from build123d import *

# Parameters (mm, degrees)
CROQUIS1_R              = 6.35
SALIENTE_EXTRUIR1_DEPTH = 6.35
CROQUIS4_W              = 4.7625
CROQUIS4_H              = 50.8
CORTAR_EXTRUIR1_DEPTH   = 3.175


with BuildPart() as part:
    # Croquis1 → Saliente-Extruir1 (new body)
    with BuildSketch(Plane(origin=(0, 0, 0), x_dir=(1, 0, 0), z_dir=(0, 1, 0))):
        with BuildLine():
            Line((35.8, -25.4), (50.8, 0))
            Line((50.8, 0), (35.8, 25.4))
            Line((35.8, 25.4), (-100, 25.4))
            Line((-100, 25.4), (-144.746813481, 47.731727951))
            ThreePointArc((-144.746813481, 47.731727951), (-149.357530471, 48.146831931), (-153.024774803, 45.321528145))
            Line((-153.024774803, 45.321528145), (-165, 25.4))
            Line((-165, 25.4), (-165, -25.4))
            Line((-165, -25.4), (-214.07384035, -47.316891892))
            Line((-214.07384035, -47.316891892), (-147.685890016, -48.399156383))
            ThreePointArc((-147.685890016, -48.399156383), (-146.176180179, -48.24234101), (-144.746813481, -47.731727951))
            Line((-144.746813481, -47.731727951), (-100, -25.4))
            Line((-100, -25.4), (35.8, -25.4))
        make_face()
        with Locations(Location((0, 0, 0), (0, 0, 270))):
            Circle(CROQUIS1_R, mode=Mode.SUBTRACT)
        with Locations(Location((-150, 0, 0), (0, 0, 270))):
            Circle(CROQUIS1_R, mode=Mode.SUBTRACT)
        with BuildLine():
            Line((-118.545100716, 27.558404082), (-142.329198773, 39.428299747))
            ThreePointArc((-142.329198773, 39.428299747), (-146.939915763, 39.843403727), (-150.607160095, 37.018099941))
            Line((-150.607160095, 37.018099941), (-157.742389512, 25.148204276))
            ThreePointArc((-157.742389512, 25.148204276), (-157.827056347, 18.750312726), (-152.3, 15.526676131))
            Line((-152.3, 15.526676131), (-121.380672526, 15.526676131))
            ThreePointArc((-121.380672526, 15.526676131), (-115.199998109, 20.420048603), (-118.545100716, 27.558404082))
        make_face(mode=Mode.SUBTRACT)
        with BuildLine():
            Line((-118.545100716, -27.558404082), (-142.329198773, -39.428299747))
            ThreePointArc((-142.329198773, -39.428299747), (-146.939915763, -39.843403727), (-150.607160095, -37.018099941))
            Line((-150.607160095, -37.018099941), (-157.742389512, -25.148204276))
            ThreePointArc((-157.742389512, -25.148204276), (-157.827056347, -18.750312726), (-152.3, -15.526676131))
            Line((-152.3, -15.526676131), (-121.380672526, -15.526676131))
            ThreePointArc((-121.380672526, -15.526676131), (-115.199998109, -20.420048603), (-118.545100716, -27.558404082))
        make_face(mode=Mode.SUBTRACT)
        with BuildLine():
            Line((-130, 6.35), (-110, 6.35))
            ThreePointArc((-110, 6.35), (-103.65, 0), (-110, -6.35))
            Line((-110, -6.35), (-130, -6.35))
            ThreePointArc((-130, -6.35), (-136.35, 0), (-130, 6.35))
        make_face(mode=Mode.SUBTRACT)
        with BuildLine():
            Line((-56.70082756, -7.67562673), (-77.066937646, 8.064222026))
            ThreePointArc((-77.066937646, 8.064222026), (-83.748665223, 8.739846385), (-87.3, 3.039848756))
            Line((-87.3, 3.039848756), (-87.3, -12.7))
            ThreePointArc((-87.3, -12.7), (-85.440128061, -17.190128061), (-80.95, -19.05))
            Line((-80.95, -19.05), (-60.583889913, -19.05))
            ThreePointArc((-60.583889913, -19.05), (-54.57442778, -14.751551819), (-56.70082756, -7.67562673))
        make_face(mode=Mode.SUBTRACT)
        with BuildLine():
            Line((-57.963298738, 19.05), (-38.1, 19.05))
            ThreePointArc((-38.1, 19.05), (-33.609871939, 17.190128061), (-31.75, 12.7))
            Line((-31.75, 12.7), (-31.75, -2.651253459))
            ThreePointArc((-31.75, -2.651253459), (-35.301334777, -8.351251089), (-41.983062354, -7.67562673))
            Line((-41.983062354, -7.67562673), (-61.846361092, 7.67562673))
            ThreePointArc((-61.846361092, 7.67562673), (-63.972760872, 14.751551819), (-57.963298738, 19.05))
        make_face(mode=Mode.SUBTRACT)
    extrude(amount=SALIENTE_EXTRUIR1_DEPTH)

    # Croquis4 → Cortar-Extruir1 (cut)
    with BuildSketch(Plane(origin=(0, 6.35, 0), x_dir=(1, 0, 0), z_dir=(0, 1, 0))):
        with Locations((-97.61875, 0)):
            Rectangle(CROQUIS4_W, CROQUIS4_H)
        with Locations((33.41875, 0)):
            Rectangle(CROQUIS4_W, CROQUIS4_H)
    extrude(amount=-CORTAR_EXTRUIR1_DEPTH, mode=Mode.SUBTRACT)


solid = part.part
Could you check a few things on this model? Use its own coordinates, in mm. A direction names the side the tool comes from. Give positions to 0.01 mm unless a question says otherwise; leave off trailing zeros. Order: outer loops, then holes, each group sorted by start corner. A loop starts at its lowest first (then second) coordinate and runs counter-clockwise, first axis right, second up. Notation, with made-up numbers: (-28, 37) -> (-9, 37) arc R19 ccw to (-9, 65) -> close; hole circle Ø9 at (11, -24). An arc over 180 degrees is marked (long way). Return JSON: item names as keys, results as strings.
1. Thinking about a two-plate mould opening in X: for faces 1 (the flat face through (-158.93, 3.13, -35.5)), 2 (the cylindrical face through (-149.294, 3.131, -48.165)), 3 (the cylindrical face through (-136.35, 3.13, 0.14)), which applies, pulls with the +X half, pulls with the -X half, needs draft (parallel to the pull), parting line crosses it, or undercut?
Answer list:
{"face 1": "pulls with the -X half", "face 2": "parting line crosses it", "face 3": "undercut"}
2. Imagine slicing it at B-B on x = -92. List the corners of the cut face in (y, z) for me.
Answer list:
{"outline": "(0, -25.4) -> (6.35, -25.4) -> (6.35, 25.4) -> (0, 25.4) -> close"}
3. Imagine slicing it at D-D on z = -31. List the corners of the cut face in (x, y) for me, then the cut area to 3 significant figures.
Answer list:
{"outline": "(-161.63, 0) -> (-154.22, 0) -> (-154.22, 6.35) -> (-161.63, 6.35) -> close; (-125.44, 0) -> (-111.22, 0) -> (-111.22, 6.35) -> (-125.44, 6.35) -> close", "area": "137 mm2"}
4. Imagine slicing it at C-C on y = 1.5. Give the number of separate pieces and of enclosed holes in the cut face, then the cut area to 3 significant figures.
Answer list:
{"separate pieces": "1", "enclosed holes": "7", "area": "9,400 mm2"}
5. On a 3-axis mill with a long thin cutter (end or side, diameter ignored), from which of +Z, -Z, +X, -X, +Y, -Y can I reach the whole of each face in a straight line? I mean faces 4 (the cylindrical face through (-33.66, 3.13, -17.24)), 5 (the flat face through (-31, 3, -25.4)), 6 (the flat face through (-33, 3, 25.4)). Say none if no direction works.
Answer list:
{"face 4": "+Y, -Y", "face 5": "-Z, +X, +Y, -Y", "face 6": "+Z, +X, +Y, -Y"}
6. Imagine slicing it at A-A on z = 34. List the corners of the cut face in (x, y) for me.
Answer list:
{"outline": "(-184.26, 0) -> (-152.42, 0) -> (-152.42, 6.35) -> (-184.26, 6.35) -> close; (-131.45, 0) -> (-117.23, 0) -> (-117.23, 6.35) -> (-131.45, 6.35) -> close"}
7. I need wall thicknesses on line 1 (Z direction, x = -139.5, y = 5); line 2 (Z direction, x = -154, y = 0.5); line 3 (Z direction, x = -55, y = 4.25). Which ranges of each line are inside material? Lowest first, please. Write a range as from..to.
Answer list:
{"line 1": "z = -45.11..-38.02, -15.53..15.53, 38.02..45.11", "line 2": "z = -43.7..-31.37, -15.76..-4.93, 4.93..15.76, 31.37..48.3", "line 3": "z = -25.4..-19.05, -2.38..9.68, 15.72..25.4"}
8. For pin 1 Ø3 at (y, z) = (5.5, 6) entering from +X; pin 2 Ø1.9 at (x, y) = (-45.5, 2.5) entering from +Z; pin 3 Ø1 at (x, y) = (-15.5, 4) entering from -Z; pin 4 Ø10 at (x, z) = (-150, 0) entering from -Y, each with a flat end and sliding along its axis, tell me the tip position at first contact or that it passes through.
Answer list:
{"pin 1": "stops at x = 48.14", "pin 2": "stops at z = 25.4", "pin 3": "stops at z = -25.4", "pin 4": "passes through"}
